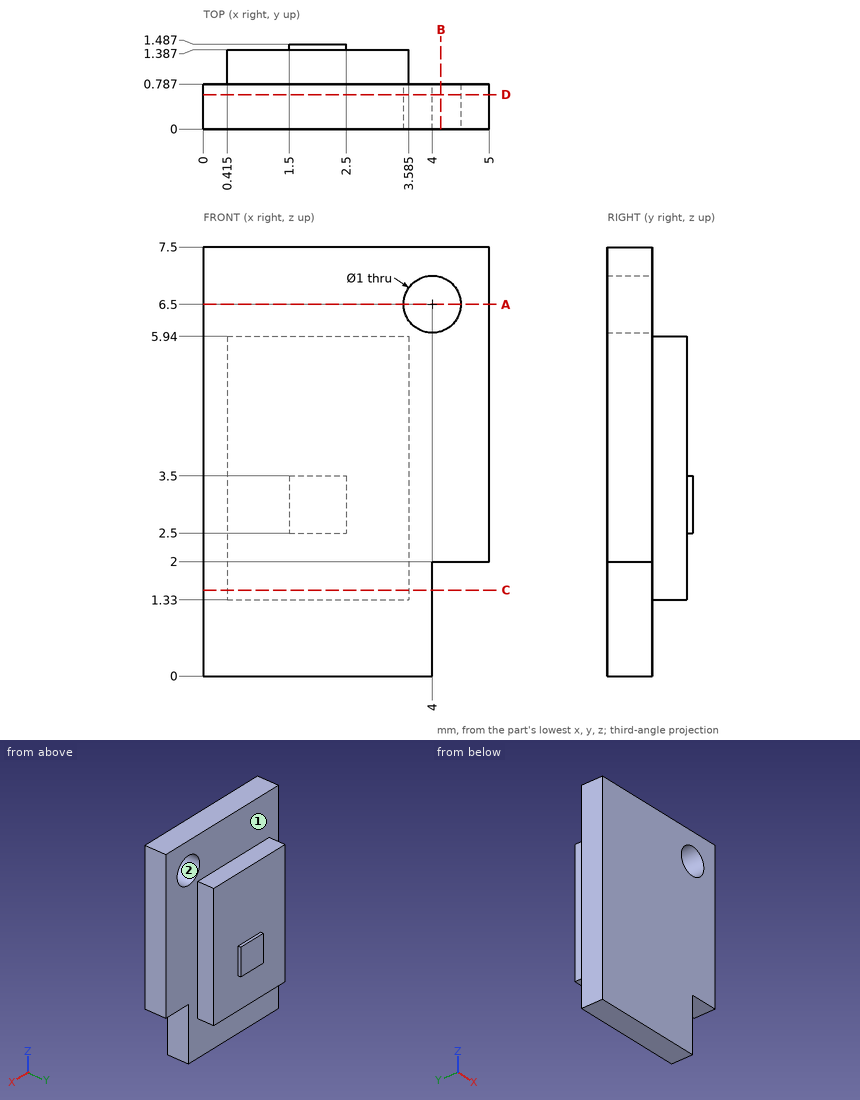
Verification items for this drawing (mm, ordinates from the low corner). Coordinates: 2 decimals unless noted, no trailing zeros. Order: outer loops, then holes, each group sorted by start corner. A loop starts at its lowest first (then second) coordinate and runs counter-clockwise, first axis right, second up. Notation, with made-up numbers: (-8, 31) - (42, 31) arc R4 ccw to (42, 37) - close; hole circle Ø11 at (7.5, -29.75). An arc over 180 degrees is marked (long way). Answer in a Markdown table with one row per item. Add a question column.
1. Section check D-D (y = 0.6). Enter the section's corners in (x, z).
2. Draft check along Z on the marked faces 1 and 2. Enter one of: +Z half, -Z half, draft (parallel to the pull), parting line (faces both ways), or undercut.
3. Gauge pin test, flat ends, axial feed: pin 1 Ø1 at (x, z) = (2.5, 6) entering from +Y; pin 2 Ø0.6 at (x, y) = (4.5, 0.5) entering from -Z; pin 3 Ø0.7 at (x, y) = (2, 1) entering from +Z. Record the tip position at first contact, or that the pin passes through.
4. Section check C-C (z = 1.5). Enter the section's corners in (x, y) (1 decimal).
5. Section check A-A (z = 6.5). Enter the section's corners in (x, y).
6. Section check B-B (x = 4.15). Enter the section's corners in (y, z).
7. Material ranges on L1, parallel to X at y = 0.25, z = 6.5; L2, parallel to Z at x = 2.9, y = 1.05; L3, parallel to Y at x = 0.35, z = 4.75, recorded low to high. Write a range as [from, to].
Data:
| question | item | result |
|---|---|---|
| 1 | outline | (0, 0) - (4, 0) - (4, 2) - (5, 2) - (5, 7.5) - (0, 7.5) - close; hole circle Ø1 at (4, 6.5) |
| 2 | face 1 | draft |
| 2 | face 2 | undercut |
| 3 | pin 1 | stops at y = 1.39 |
| 3 | pin 2 | stops at z = 2 |
| 3 | pin 3 | stops at z = 7.5 |
| 4 | outline | (0, 0) - (4, 0) - (4, 0.8) - (3.6, 0.8) - (3.6, 1.4) - (0.4, 1.4) - (0.4, 0.8) - (0, 0.8) - close |
| 5 | outline | (0, 0) - (3.5, 0) - (3.5, 0.79) - (0, 0.79) - close; (4.5, 0) - (5, 0) - (5, 0.79) - (4.5, 0.79) - close |
| 6 | outline | (0, 2) - (0.79, 2) - (0.79, 6.02) - (0, 6.02) - close; (0, 6.98) - (0.79, 6.98) - (0.79, 7.5) - (0, 7.5) - close |
| 7 | L1 | x = [0, 3.5], [4.5, 5] |
| 7 | L2 | z = [1.33, 5.94] |
| 7 | L3 | y = [0, 0.79] |
